Read the model definition and answer for the solid it produces. Units are mm, in the model's axes. A direction names the side the tool comes from. Coordinates: 2 decimals unless noted, no trailing zeros. Order: outer loops, then holes, each group sorted by start corner. A loop starts at its lowest first (then second) coordinate and runs counter-clockwise, first axis right, second up. Notation, with made-up numbers: M -9.5,68 L 11.5,68 A19 cw 11.5,78 Z; hole C 84.25,73.5 d1. An arc over 180 degrees is marked long. Use a Markdown table: item, result. Add a question column.
1) Find section A-A on y = 20. Write down the section's boundary in (x, z).
2) Find the intervals of material crossed by probe 1 along Y at (x, z) = (-10, 0.85); probe 2 along X at (y, z) = (20, 2.5); probe 3 along X at (y, z) = (-9.5, 29), in increasing order. Write a range as [from, to].
3) Each of these flat-tipped pins is pushed along its axis until it touches: pin 1 Ø1 at (y, z) = (9, 50.5) entering from -X; pin 2 Ø1 at (x, y) = (-7.5, 5.5) entering from +Z. Where does it stop, or does it pass through?
4) For faces 1 (the face through (11.75, 0, 44)), 2 (the face through (10, 0, 33)), 3 (the face through (12, 0, 63.5)), determine the directions among +Z, -Z, +X, -X, +Y, -Y from which every point of the face is accessible in a straight line to the end or side of a thin tool.
5) Find section D-D on y = -13.5. Write down the section's boundary in (x, z).
6) Find section C-C on x = -10. Write down the section's boundary in (y, z), plus the area to 3 significant figures.
7) The mould has two halves that part along Z. Classify faces 4 (the face through (13.4, -0.3, 50.1)), 5 (the face through (0, 0, 0)), 6 (the face through (-15, 0, 2)): released by +Z, released by -Z, zero draft, split by the parting line, or undercut.
8) Find section B-B on z = 49.5. Write down the section's boundary in (x, y).
from build123d import *

# Parameters (mm, degrees)
SKETCH_2_W          = 30
SKETCH_2_H          = 50
SKETCH_2_R          = 2.1
EXTRUDE_1_DEPTH     = 3.5
SKETCH_3_W          = 5
SKETCH_3_H          = 50
EXTRUDE_2_DEPTH     = 60
CUT_EXTRUDE_1_REACH = 84.202


with BuildPart() as part:
    # 草图2 → 凸台-拉伸1 (new body)
    with BuildSketch(Plane.XY):
        Rectangle(SKETCH_2_W, SKETCH_2_H)
        with Locations((-10, -20)):
            Circle(SKETCH_2_R, mode=Mode.SUBTRACT)
        with Locations(Location((-10, 20, 0), (0, 0, 180))):
            Circle(SKETCH_2_R, mode=Mode.SUBTRACT)
    extrude(amount=EXTRUDE_1_DEPTH)

    # 草图3 → 凸台-拉伸2 (add)
    with BuildSketch(Plane.XY.offset(3.5)):
        with Locations((12.5, 0)):
            Rectangle(SKETCH_3_W, SKETCH_3_H)
    extrude(amount=EXTRUDE_2_DEPTH)

    # 草图6 → 切除-拉伸1 (cut, up to next)
    with BuildSketch(Plane.XZ.offset(25), mode=Mode.PRIVATE) as cut_extrude_1_sk1:
        Polygon((15, 48.5), (11.75, 51.75), (11.75, 35.75), (15, 39), align=None)
    cut_extrude_1_tool1 = extrude(cut_extrude_1_sk1.sketch, amount=-CUT_EXTRUDE_1_REACH, mode=Mode.PRIVATE) & part.part
    add(cut_extrude_1_tool1.solids().sort_by_distance((13.236928, -25, 43.75))[0], mode=Mode.SUBTRACT)


solid = part.part
Check result:
| question | item | result |
|---|---|---|
| 1 | outline | M -15,0 L -12.1,0 L -12.1,3.5 L -15,3.5 Z; M -7.9,0 L 15,0 L 15,39 L 11.75,35.75 L 11.75,51.75 L 15,48.5 L 15,63.5 L 10,63.5 L 10,3.5 L -7.9,3.5 Z |
| 2 | probe 1 | y = [-25, -22.1], [-17.9, 17.9], [22.1, 25] |
| 2 | probe 2 | x = [-15, -12.1], [-7.9, 15] |
| 2 | probe 3 | x = [10, 15] |
| 3 | pin 1 | stops at x = 10 |
| 3 | pin 2 | stops at z = 3.5 |
| 4 | face 1 | +Y, -Y |
| 4 | face 2 | +Z, -X, +Y, -Y |
| 4 | face 3 | +Z, +X, -X, +Y, -Y |
| 5 | outline | M -15,0 L 15,0 L 15,39 L 11.75,35.75 L 11.75,51.75 L 15,48.5 L 15,63.5 L 10,63.5 L 10,3.5 L -15,3.5 Z |
| 6 | outline | M -25,0 L -22.1,0 L -22.1,3.5 L -25,3.5 Z; M -17.9,0 L 17.9,0 L 17.9,3.5 L -17.9,3.5 Z; M 22.1,0 L 25,0 L 25,3.5 L 22.1,3.5 Z |
| 6 | area | 146 mm2 |
| 7 | face 4 | undercut |
| 7 | face 5 | released by -Z |
| 7 | face 6 | zero draft |
| 8 | outline | M 10,-25 L 11.75,-25 L 11.75,25 L 10,25 Z; M 14,-25 L 15,-25 L 15,25 L 14,25 Z |
